Can you work these out from the model? Positions are in its coordinate system, mm. A direction names the side the tool comes from. Coordinates: 2 decimals unless noted, no trailing zeros. Order: outer loops, then holes, each group sorted by start corner. A loop starts at its lowest first (then second) coordinate and runs counter-clockwise, first axis right, second up. Notation, with made-up numbers: (16, 52.5) - (34, 52.5) arc R20 ccw to (34, 63.5) - close; hole circle Ø8 at (15, -36.75). An arc over 180 degrees is marked (long way). Use a Markdown table: item, result. Add a question column.
(1) I want a section at C-C (z = -24). List the corners of the cut face in (x, y) for me, and give its area (3 significant figures).
(2) If I drill on L1, parallel to X at y = 1, z = 0; L2, parallel to X at y = -3.75, z = 0; L3, parallel to Z at x = 232, y = -1, over which ranges is the centre line in solid material (lowest first)? Write a range as [from, to].
(3) On a 3-axis mill with a long thin cutter (end or side, diameter ignored), from which of +Z, -Z, +X, -X, +Y, -Y can I reach the whole of each face in a straight line? I mean faces 1 (the cylindrical face through (-239.13, 18.49, 1.55)), 2 (the flat face through (-226, 0, 6)). Say none if no direction works.
(4) I want a section at A-A (z = 0). List the corners of the cut face in (x, y) for me, and give its area (3 significant figures).
(5) For pin 1 Ø3 at (y, z) = (6.5, 11.5) entering from +X; pin 2 Ø12 at (x, z) = (202, 17.5) entering from +Y; pin 3 Ø6 at (y, z) = (11.5, 13.5) entering from -X, each with a flat end and sliding along its axis, tell me the tip position at first contact or that it passes through.
(6) I want a section at B-B (x = -210.5). List the corners of the cut face in (y, z) for me.
(7) I want a section at D-D (x = 67). List the corners of the cut face in (y, z) for me, and give its area (3 significant figures).
```python
from build123d import *

# Parameters (mm, degrees)
BOSS_EXTRU_1_DEPTH      = 8
ESQUISSE2_R             = 7.15
ENL_V_MAT_EXTRU_1_DEPTH = 265.732643435
R_VOLUTION1_ANGLE       = 180
ESQUISSE4_R             = 7.15
ENL_V_MAT_EXTRU_2_DEPTH = 269.282863784
ESQUISSE5_R             = 30.35
ENL_V_MAT_EXTRU_6_DEPTH = 8


with BuildPart() as part:
    # Esquisse1 → Boss.-Extru.1 (new, symmetric)
    with BuildSketch(Plane(origin=(0, 0, 0), x_dir=(1, 0, 0), z_dir=(0, 1, 0))):
        with BuildLine():
            Line((-232.15, 30.35), (232.15, 30.35))
            ThreePointArc((232.15, 30.35), (262.5, 0), (232.15, -30.35))
            Line((232.15, -30.35), (-232.15, -30.35))
            ThreePointArc((-232.15, -30.35), (-262.5, 0), (-232.15, 30.35))
        make_face()
    extrude(amount=BOSS_EXTRU_1_DEPTH, both=True)

    # Esquisse2 → Enlèv. mat.-Extru.1 (cut, through all)
    with BuildSketch(Plane(origin=(0, 8, 0), x_dir=(1, 0, 0), z_dir=(0, 1, 0))):
        with Locations(Location((232.15, 0, 0), (0, 0, 270))):
            Circle(ESQUISSE2_R)
    extrude(amount=-ENL_V_MAT_EXTRU_1_DEPTH, mode=Mode.SUBTRACT)

    # Esquisse3 → Révolution1 (revolve)
    with BuildSketch(Plane(origin=(0, 8, 0), x_dir=(1, 0, 0), z_dir=(0, 1, 0))):
        with BuildLine():
            Line((-232.15, 30.35), (-232.15, -30.35))
            ThreePointArc((-232.15, -30.35), (-262.5, 0), (-232.15, 30.35))
        make_face()
    revolve(axis=Axis((-232.15, 8, -30.35), (0, 0, -1)), revolution_arc=R_VOLUTION1_ANGLE)

    # Esquisse4 → Enlèv. mat.-Extru.2 (cut, through all)
    with BuildSketch(Plane.XZ.offset(8)):
        with Locations(Location((-232.15, 0, 0), (0, 0, 270))):
            Circle(ESQUISSE4_R)
    extrude(amount=-ENL_V_MAT_EXTRU_2_DEPTH, mode=Mode.SUBTRACT)

    # Esquisse5 → Enlèv. mat.-Extru.6 (cut)
    with BuildSketch(Plane(origin=(0, 0, 0), x_dir=(1, 0, 0), z_dir=(0, 1, 0))):
        with Locations((-232.15, 0)):
            Circle(ESQUISSE5_R)
    extrude(amount=-ENL_V_MAT_EXTRU_6_DEPTH, mode=Mode.SUBTRACT)


solid = part.part
```
Answers follow:
| question | item | result |
|---|---|---|
| 1 | outline | (-250.73, 0) - (-213.57, 0) - (-213.57, -8) - (250.73, -8) - (250.73, 8) - (-213.57, 8) arc R18.58 ccw to (-250.73, 8) - close |
| 1 | area | 8,270 mm² |
| 2 | L1 | x = [-262.5, -239.3], [-225, 225], [239.3, 262.5] |
| 2 | L2 | x = [-201.8, 225], [239.3, 262.5] |
| 2 | L3 | z = [-30.35, -7.15], [7.15, 30.35] |
| 3 | face 1 | +Y, -Y |
| 3 | face 2 | -X, -Y |
| 4 | outline | (-262.5, 0) - (-239.3, 0) - (-239.3, 37.5) arc R30.35 ccw to (-262.5, 8) - close; (-225, 0) - (-201.8, 0) - (-201.8, -8) - (225, -8) - (225, 8) - (-201.8, 8) arc R30.35 ccw to (-225, 37.5) - close; (239.3, -8) - (262.5, -8) - (262.5, 8) - (239.3, 8) - close |
| 4 | area | 8,590 mm² |
| 5 | pin 1 | stops at x = 260.81 |
| 5 | pin 2 | stops at y = 8 |
| 5 | pin 3 | stops at x = -260.46 |
| 6 | outline | (-8, -30.35) - (8, -30.35) - (8, -21.27) arc R21.27 ccw to (8, 21.27) - (8, 30.35) - (-8, 30.35) - (-8, 21.27) - (0, 21.27) - (0, -21.27) - (-8, -21.27) - close |
| 7 | outline | (-8, -30.35) - (8, -30.35) - (8, 30.35) - (-8, 30.35) - close |
| 7 | area | 971 mm² |
